Check sheet for the modelled part. Datum: model origin and axes. Units: mm. A direction names the side the tool comes from. Round coordinates to 2 decimals unless told otherwise and drop trailing zeros. Order: outer loops, then holes, each group sorted by start corner. A loop starts at its lowest first (then second) coordinate and runs counter-clockwise, first axis right, second up. Notation, with made-up numbers: (4, 26) -> (38, 26) arc R22 ccw to (38, 38) -> close; hole circle Ø9 at (76.5, 4.5). An arc over 180 degrees is marked (long way). Answer in a Markdown table with one row per item.
from build123d import *

# Parameters (mm, degrees)
F0_R     = 228.6
F1_DEPTH = 6.35
F3_DEPTH = 6.351
F4_R     = 12.7
F5_DEPTH = 6.351


# Not quite as in the source:
# - ends of sketch curves that miss each other by under 0.0002 mm in the source are joined


with BuildPart() as f1:
    # F0 (on Front) → F1 (new body)
    with BuildSketch(Plane.XZ):
        Circle(F0_R)
    extrude(amount=F1_DEPTH)

    # F2 (on face) → F3 (cut, through all)
    with BuildSketch(Plane(origin=(0, 0, 0), x_dir=(-1, 0, 0), z_dir=(0, 1, 0))):
        with BuildLine():
            Line((4.4618826202, 41.03312384), (22.1427530806, 34.8808349771))
            ThreePointArc((22.1427530806, 34.8808349771), (24.1653047772, 35.8628309135), (23.1774067066, 37.8825063297))
            Line((23.1774067066, 37.8825063297), (5.5701325615, 43.8941330325))
            Line((5.5701325615, 43.8941330325), (4.6801519701, 44.1979978468))
            ThreePointArc((4.6801519701, 44.1979978468), (3.5809145294, 43.7979774539), (3.0541190675, 42.7535519863))
            ThreePointArc((3.0541190675, 42.7535519863), (3.4066096848, 41.6058073542), (4.4618826202, 41.03312384))
        make_face()
        with BuildLine():
            Line((4.6801519701, 44.1979978468), (5.5701325615, 43.8941330325))
            ThreePointArc((5.5701325615, 43.8941330325), (5.1481595065, 44.1134796096), (4.6801519701, 44.1979978468))
        make_face()
        with BuildLine():
            Line((-31.727890274, 31.0981475896), (-30.7078696735, 31.753608073))
            ThreePointArc((-30.7078696735, 31.753608073), (-31.2829212175, 31.5270943199), (-31.727890274, 31.0981475896))
        make_face()
        with BuildLine():
            Line((-15.1702982711, 41.737979033), (-30.7078696735, 31.753608073))
            Line((-30.7078696735, 31.753608073), (-31.727890274, 31.0981475896))
            ThreePointArc((-31.727890274, 31.0981475896), (-31.5281772375, 29.050280341), (-29.4747442403, 28.9196721839))
            Line((-29.4747442403, 28.9196721839), (-13.4626581421, 39.061324038))
            ThreePointArc((-13.4626581421, 39.061324038), (-12.9781507091, 41.2534716), (-15.1702982711, 41.737979033))
        make_face()
        with BuildLine():
            Line((-40.992265014, -4.8302478058), (-38.9334293172, 13.8267433983))
            ThreePointArc((-38.9334293172, 13.8267433983), (-40.5597026781, 15.5876336173), (-42.0757424664, 13.7309907417))
            Line((-42.0757424664, 13.7309907417), (-44.151831017, -4.7859890094))
            ThreePointArc((-44.151831017, -4.7859890094), (-42.5964510469, -6.5502125075), (-40.992265014, -4.8302478058))
        make_face()
        with BuildLine():
            Line((34.8455227588, 22.1234679996), (41.0769142774, 4.4353792716))
            ThreePointArc((41.0769142774, 4.4353792716), (43.1041953835, 3.4664465633), (44.0697534768, 5.4953371086))
            Line((44.0697534768, 5.4953371086), (37.7754084063, 23.174174494))
            Line((37.7754084063, 23.174174494), (37.5676840132, 23.7576070393))
            ThreePointArc((37.5676840132, 23.7576070393), (35.3876634671, 24.3047338716), (34.8455227588, 22.1234679996))
        make_face()
        with BuildLine():
            Line((37.5676840132, 23.7576070393), (37.7754084063, 23.174174494))
            ThreePointArc((37.7754084063, 23.174174494), (37.7002728684, 23.4761185604), (37.5676840132, 23.7576070393))
        make_face()
        with BuildLine():
            Line((-23.6211183536, -37.6470325436), (-23.9224947466, -37.3484117712))
            ThreePointArc((-23.9224947466, -37.3484117712), (-23.7818274542, -37.5078355326), (-23.6211183536, -37.6470325436))
        make_face()
        with BuildLine():
            Line((-37.3220998756, -24.0713252866), (-23.9224947466, -37.3484117712))
            Line((-23.9224947466, -37.3484117712), (-23.6211183536, -37.6470325436))
            ThreePointArc((-23.6211183536, -37.6470325436), (-21.3089064889, -37.2063703199), (-21.9768545063, -34.9493031191))
            Line((-21.9768545063, -34.9493031191), (-35.0812263092, -21.8220953205))
            ThreePointArc((-35.0812263092, -21.8220953205), (-37.3262780755, -21.8262735204), (-37.3220998756, -24.0713252866))
        make_face()
        with BuildLine():
            Line((14.1274943747, -38.8257185152), (-4.6460917137, -41.0236705883))
            ThreePointArc((-4.6460917137, -41.0236705883), (-6.2226980939, -42.6185631758), (-4.6312320578, -44.1986283327))
            Line((-4.6312320578, -44.1986283327), (-4.2448360729, -44.1498861266))
            Line((-4.2448360729, -44.1498861266), (13.7359027682, -41.8816925861))
            Line((13.7359027682, -41.8816925861), (15.2375878216, -41.6922614193))
            ThreePointArc((15.2375878216, -41.6922614193), (15.7924641961, -39.8291626809), (14.1274943747, -38.8257185152))
        make_face()
        with BuildLine():
            Line((-4.2448360729, -44.1498861266), (-4.6312320578, -44.1986283327))
            ThreePointArc((-4.6312320578, -44.1986283327), (-4.4365336717, -44.1861513585), (-4.2448360729, -44.1498861266))
        make_face()
        with BuildLine():
            ThreePointArc((13.8057650277, -41.9070382349), (14.5475871245, -41.9723850949), (15.2375878216, -41.6922614193))
            Line((15.2375878216, -41.6922614193), (13.8057650277, -41.9070382349))
        make_face()
        with BuildLine():
            Line((13.8057650277, -41.9070382349), (15.2375878216, -41.6922614193))
            Line((15.2375878216, -41.6922614193), (13.7359027682, -41.8816925861))
            ThreePointArc((13.7359027682, -41.8816925861), (13.7706855601, -41.8947742862), (13.8057650277, -41.9070382349))
        make_face()
        with BuildLine():
            Line((39.1205111726, -13.2355457292), (29.0774053416, -29.3519750753))
            ThreePointArc((29.0774053416, -29.3519750753), (29.5860528198, -31.5394518473), (31.7731794636, -31.0293009591))
            Line((31.7731794636, -31.0293009591), (41.6947378015, -15.0590532006))
            Line((41.6947378015, -15.0590532006), (41.9843072327, -14.5929474337))
            ThreePointArc((41.9843072327, -14.5929474337), (41.1912924211, -12.5663543268), (39.1205111726, -13.2355457292))
        make_face()
        with BuildLine():
            Line((41.9843072327, -14.5929474337), (41.6947378015, -15.0590532006))
            ThreePointArc((41.6947378015, -15.0590532006), (41.8598142795, -14.8386066278), (41.9843072327, -14.5929474337))
        make_face()
    extrude(amount=-F3_DEPTH, mode=Mode.SUBTRACT)

    # F4 (on face) → F5 (cut, through all)
    with BuildSketch(Plane.XZ.offset(6.35)):
        Circle(F4_R)
    extrude(amount=-F5_DEPTH, mode=Mode.SUBTRACT)


solid = f1.part
Item 1: Cross-section at C-C (z = -68). Record the boundary of the cut face in (x, y), and give its area (3 significant figures).
Result sheet:
| item | result |
|---|---|
| outline | (-218.25, -6.35) -> (218.25, -6.35) -> (218.25, 0) -> (-218.25, 0) -> close |
| area | 2,770 mm^2 |
Item 2: Cross-section at B-B (x = -111). Record the boundary of the cut face in (y, z), and give its area (3 significant figures).
Result sheet:
| item | result |
|---|---|
| outline | (-6.35, -199.84) -> (0, -199.84) -> (0, 199.84) -> (-6.35, 199.84) -> close |
| area | 2,540 mm^2 |
Item 3: Depth check by flat-ended pin: P1, Ø5, axis at x = 110, z = -105.5, coming from the +Y side. Enter the tip coordinate at first touch or a pass-through.
Result sheet:
| item | result |
|---|---|
| P1 | stops at y = 0 |
Item 4: Scan lines: line 1 (Z direction, x = 4, y = -1) (3 decimals); line 2 (X direction, y = -1, z = 23); line 3 (Z direction, x = -26, y = -6). Record each from-to range of solid material in increasing order. Write a range as [from, to].
Result sheet:
| item | result |
|---|---|
| line 1 | z = [-228.565, -44.119], [-40.948, -12.054], [12.054, 228.565] |
| line 2 | x = [-227.44, -37.84], [-34.62, 227.44] |
| line 3 | z = [-227.12, 227.12] |
Item 5: Set-up check for faces 4 (the flat face through (-3, -6.35, -48)), 5 (the flat face through (28.437, -3.131, -28.478)): record each of +Z, -Z, +X, -X, +Y, -Y from which the full face is reachable in a straight line by a thin tool's end or side.
Result sheet:
| item | result |
|---|---|
| face 4 | +Z, -Z, +X, -X, -Y |
| face 5 | +Y, -Y |
Item 6: Cross-section at A-A (y = -4.5). State how many separate pieces and enclosed holes the cut face has, and give its area (3 significant figures).
Result sheet:
| item | result |
|---|---|
| separate pieces | 1 |
| enclosed holes | 8 |
| area | 163,000 mm^2 |
Item 7: Mould release check, pull along X, two halves, no side actions. Record for faces 1 (the cylindrical face through (-228.38, -3.13, 10.05)), 2 (the flat face through (22.83, -3.131, 36.816)), 3 (the flat face through (-3, 0, -48)): pulls with the +X half, pulls with the -X half, needs draft (parallel to the pull), parting line crosses it, or undercut.
Result sheet:
| item | result |
|---|---|
| face 1 | parting line crosses it |
| face 2 | undercut |
| face 3 | needs draft |
